```python
from build123d import *

# Parameters (mm, degrees)
SKETCH1_W                = 56.896
SKETCH1_H                = 27.94
BOSS_EXTRUDE1_DEPTH      = 2.54
CUT_EXTRUDE1_DEPTH       = 3.54
FILLET1_R                = 1.27
EXTRUDE_THIN1_DEPTH      = 12.7
EXTRUDE_THIN1_DEPTH_BACK = 28.448


with BuildPart() as part:
    # Sketch1 → Boss-Extrude1 (new body)
    with BuildSketch(Plane.XY):
        Rectangle(SKETCH1_W, SKETCH1_H)
    extrude(amount=BOSS_EXTRUDE1_DEPTH)

    # Sketch2 → Cut-Extrude1 (cut, through all)
    with BuildSketch(Plane.XY.offset(2.54)):
        with BuildLine():
            Line((-15.875, -13.97), (15.875, -13.97))
            ThreePointArc((15.875, -13.97), (0, -8.397868645), (-15.875, -13.97))
        make_face()
    extrude(amount=-CUT_EXTRUDE1_DEPTH, mode=Mode.SUBTRACT)

    # Fillet1
    fillet1_edges = [part.edges().sort_by_distance(p)[0] for p in [
        (-15.875, -13.97, 1.27),
        (15.875, -13.97, 1.27),
        (28.448, -13.97, 1.27),
        (-28.448, -13.97, 1.27),
        (-28.448, 13.97, 1.27),
        (28.448, 13.97, 1.27),
    ]]
    fillet(fillet1_edges, radius=FILLET1_R)

    # Sketch4 → Extrude-Thin1 (add, two sides)
    with BuildSketch(Plane(origin=(0, 0, 0), x_dir=(0, 0, -1), z_dir=(1, 0, 0))) as extrude_thin1_sk:
        Polygon((0, -4.064), (7.112, -4.064), (7.112, 4.064), (0, 4.064), (0, 6.604), (9.652, 6.604), (9.652, -6.604), (0, -6.604), align=None)
    extrude(amount=EXTRUDE_THIN1_DEPTH)
    extrude(extrude_thin1_sk.sketch, amount=-EXTRUDE_THIN1_DEPTH_BACK)


solid = part.part
```
Part model, mm, in its own coordinate system. A direction names the side the tool comes from. Round coordinates to 2 decimals unless told otherwise and drop trailing zeros. Write each loop counter-clockwise with the first axis right and the second up, starting at its lowest first coordinate (ties: lowest second). Pieces come first, ordered by that corner, then holes.
Item 1: Drop flat-ended pins along their axis: pin 1 Ø5 at (y, z) = (-0.5, -5.5) entering from +X; pin 2 Ø5.5 at (x, z) = (-11.5, -4.5) entering from -Y; pin 3 Ø5.5 at (x, z) = (-5.5, -3.5) entering from +Y. Give the stop position or say it passes through.
Results:
pin 1: stops at x = 12.7
pin 2: stops at y = -6.6
pin 3: stops at y = 6.6
Item 2: Which spindle directions (+Z, -Z, +X, -X, +Y, -Y) get a long thin tool onto all of the face, cutting with end or side? Do faces 4 (the flat face through (-8, 0, -7.112)), 5 (the flat face through (-8, 6.604, -5)), 6 (the flat face through (12.7, 0, -8)), 7 (the flat face through (-8, -6.604, -5)), 8 (the cylindrical face through (0.2, -8.4, 1.3)). Say none if no direction does.
Results:
face 4: +X, -X
face 5: -Z, +X, -X, +Y
face 6: -Z, +X, +Y, -Y
face 7: -Z, +X, -X, -Y
face 8: +Z, -Z, -Y
Item 3: Cut at B-B, the plane z = -5. Give the cut face in (x, y), plus the area to 3 significant figures.
Results:
outline: (-28.45, -6.6) - (12.7, -6.6) - (12.7, -4.06) - (-28.45, -4.06) - close; (-28.45, 4.06) - (12.7, 4.06) - (12.7, 6.6) - (-28.45, 6.6) - close
area: 209 mm2
Item 4: Cut at A-A, the plane y = 0.5. Give the cut face in (x, z).
Results:
outline: (-28.45, -9.65) - (12.7, -9.65) - (12.7, -7.11) - (-28.45, -7.11) - close; (-28.45, 0) - (28.45, 0) - (28.45, 2.54) - (-28.45, 2.54) - close
Item 5: Cut at D-D, the plane y = 10.25. Give the cut face in (x, z).
Results:
outline: (-28.45, 0) - (28.45, 0) - (28.45, 2.54) - (-28.45, 2.54) - close
Item 6: Two-plate mould, pull along Y, no slides. Class faces 1 (the cylindrical face through (-28.086, 13.588, 1.288)), 2 (the cylindrical face through (-28.086, -13.588, 1.288)), 3 (the flat face through (-8, -4.064, -4)): +Y half, -Y half, draft (parallel to the pull), parting line (faces both ways), or undercut.
Results:
face 1: +Y half
face 2: -Y half
face 3: undercut
Item 7: Cut at C-C, the plane x = -7.5. Give the cut face in (y, z).
Results:
outline: (-9.53, 0) - (-6.6, 0) - (-6.6, -9.65) - (6.6, -9.65) - (6.6, 0) - (13.97, 0) - (13.97, 2.54) - (-9.53, 2.54) - close; hole (-4.06, -7.11) - (4.06, -7.11) - (4.06, 0) - (-4.06, 0) - close
Item 8: Probe L1, parallel to Z at x = 3.5, y = 1.25; L2, parallel to Y at x = 5, z = -2.5; L3, parallel to Z at x = 25, y = -1. List the from-to ranges inside material, lowest first.
Results:
L1: z = -9.65 to -7.11, 0 to 2.54
L2: y = -6.6 to -4.06, 4.06 to 6.6
L3: z = 0 to 2.54
